Design review of the part built by this model. Coordinates are the model's own, in mm. A direction names the side the tool comes from. Give positions to 0.01 mm unless a question says otherwise; leave off trailing zeros. Write each loop counter-clockwise with the first axis right and the second up, starting at its lowest first coordinate (ties: lowest second). Pieces come first, ordered by that corner, then holes. Notation, with made-up numbers: M 17.5,-5 L 51.5,-5 A8 ccw 51.5,0 Z; hole C 66.25,75 d6. An arc over 180 degrees is marked long. Use a Markdown table: item, result. Add a question column.
```python
from build123d import *

# Parameters (mm, degrees)
SKETCH1_W                = 10
SKETCH1_H                = 20
BOSS_EXTRUDE2_DEPTH      = 10
SKETCH3_W                = 10
SKETCH3_H                = 20
BOSS_EXTRUDE3_DEPTH      = 10
SKETCH4_W                = 62.5
SKETCH4_H                = 5
BOSS_EXTRUDE4_DEPTH      = 10
SKETCH6_R                = 1
CUT_EXTRUDE1_DEPTH       = 10
CUT_EXTRUDE3_START       = -10
SKETCH10_R               = 1
CUT_EXTRUDE3_DEPTH       = 10
SKETCH11_W               = 50
SKETCH11_H               = 50
BOSS_EXTRUDE8_DEPTH      = 10
SKETCH18_W               = 10
SKETCH18_H               = 10
BOSS_EXTRUDE9_DEPTH      = 6
SKETCH20_W               = 10
SKETCH20_H               = 10
BOSS_EXTRUDE10_DEPTH     = 12
SKETCH23_W               = 28.6
SKETCH23_H               = 45
CUT_EXTRUDE10_DEPTH      = 7.5
SKETCH24_W               = 6.4
SKETCH24_H               = 7.5
CUT_EXTRUDE11_DEPTH      = 4.1
SKETCH25_W               = 2.3
SKETCH25_H               = 2.5
CUT_EXTRUDE12_DEPTH      = 41
SKETCH26_W               = 2.3
SKETCH26_H               = 2.4
CUT_EXTRUDE13_DEPTH      = 41
SKETCH27_R               = 1
CUT_EXTRUDE14_DEPTH      = 10
SKETCH28_R               = 1
CUT_EXTRUDE15_DEPTH      = 10
SKETCH31_W               = 12.5
SKETCH31_H               = 10
BOSS_EXTRUDE11_DEPTH     = 5
SKETCH32_W               = 10
SKETCH32_H               = 10
CUT_EXTRUDE16_DEPTH      = 7.5
CUT_EXTRUDE17_DEPTH      = 7.5
SKETCH33_W               = 10
SKETCH33_H               = 10
BOSS_EXTRUDE12_DEPTH     = 5
SKETCH34_W               = 10
SKETCH34_H               = 10
BOSS_EXTRUDE13_DEPTH     = 5
SKETCH35_W               = 10
SKETCH35_H               = 10
BOSS_EXTRUDE14_DEPTH     = 3.5
SKETCH36_W               = 10
SKETCH36_H               = 10
BOSS_EXTRUDE15_DEPTH     = 9.5
CUT_EXTRUDE18_DEPTH      = 90.5
CUT_EXTRUDE18_DEPTH_BACK = 15.5
SKETCH37_R               = 1.25
CUT_EXTRUDE19_DEPTH      = 88.5
CUT_EXTRUDE19_DEPTH_BACK = 15.5
SKETCH38_R               = 1.25
SKETCH39_W               = 29.967126749
SKETCH39_H               = 31.835751001
SKETCH39_W_2             = 15.617210398
SKETCH39_H_2             = 32.298255859
CUT_EXTRUDE20_DEPTH      = 36
SKETCH40_W               = 10
SKETCH40_H               = 50
BOSS_EXTRUDE16_DEPTH     = 11
SKETCH41_W               = 4
SKETCH41_H               = 10
BOSS_EXTRUDE17_DEPTH     = 10
SKETCH42_R               = 1.5
CUT_EXTRUDE21_DEPTH      = 80


with BuildPart() as part:
    # Sketch1 → Boss-Extrude2 (new body)
    with BuildSketch(Plane(origin=(0, 0, 0), x_dir=(1, 0, 0), z_dir=(0, 1, 0))):
        with Locations((5, 10)):
            Rectangle(SKETCH1_W, SKETCH1_H)
    extrude(amount=BOSS_EXTRUDE2_DEPTH)



with BuildPart() as body_2:
    # Sketch3 → Boss-Extrude3 (new body)
    with BuildSketch(Plane(origin=(0, 0, 0), x_dir=(1, 0, 0), z_dir=(0, 1, 0))):
        with Locations((77.5, 10)):
            Rectangle(SKETCH3_W, SKETCH3_H)
    extrude(amount=BOSS_EXTRUDE3_DEPTH)


with BuildPart() as part_1:
    add(part.part)

    add(body_2.part)  # Boss-Extrude4 merges body 2
    # Sketch4 → Boss-Extrude4 (add)
    with BuildSketch(Plane(origin=(0, 0, 0), x_dir=(1, 0, 0), z_dir=(0, 1, 0))):
        with Locations((41.25, 10)):
            Rectangle(SKETCH4_W, SKETCH4_H)
    extrude(amount=BOSS_EXTRUDE4_DEPTH)

    # Sketch6 → Cut-Extrude1 (cut)
    with BuildSketch(Plane(origin=(10, 0, 0), x_dir=(0, 0, -1), z_dir=(1, 0, 0))):
        with Locations((16.25, 5)):
            Circle(SKETCH6_R)
    extrude(amount=-CUT_EXTRUDE1_DEPTH, mode=Mode.SUBTRACT)

    # Sketch10 → Cut-Extrude3 (cut)
    with BuildSketch(Plane.ZY.offset(-72.5).offset(CUT_EXTRUDE3_START)):
        with Locations(Location((-16.25, 5, 0), (0, 0, 180))):
            Circle(SKETCH10_R)
    extrude(amount=CUT_EXTRUDE3_DEPTH, mode=Mode.SUBTRACT)

    # Sketch11 → Boss-Extrude8 (add)
    with BuildSketch(Plane(origin=(0, 0, -12.5), x_dir=(-1, 0, 0), z_dir=(0, 0, -1))):
        with Locations((-35, 20)):
            Rectangle(SKETCH11_W, SKETCH11_H)
    extrude(amount=-BOSS_EXTRUDE8_DEPTH)

    # Sketch18 → Boss-Extrude9 (add)
    with BuildSketch(Plane.XY):
        with Locations((5, 5)):
            Rectangle(SKETCH18_W, SKETCH18_H)
    extrude(amount=BOSS_EXTRUDE9_DEPTH)

    # Sketch20 → Boss-Extrude10 (add)
    with BuildSketch(Plane.XZ):
        with Locations((77.5, -7.5)):
            Rectangle(SKETCH20_W, SKETCH20_H)
        with Locations((5, -7.5)):
            Rectangle(SKETCH20_W, SKETCH20_H)
    extrude(amount=BOSS_EXTRUDE10_DEPTH)

    # Sketch23 → Cut-Extrude10 (cut)
    with BuildSketch(Plane(origin=(0, 0, -12.5), x_dir=(-1, 0, 0), z_dir=(0, 0, -1))):
        with Locations((-35, 22.5)):
            Rectangle(SKETCH23_W, SKETCH23_H)
    extrude(amount=-CUT_EXTRUDE10_DEPTH, mode=Mode.SUBTRACT)

    # Sketch24 → Cut-Extrude11 (cut)
    with BuildSketch(Plane(origin=(0, 45, 0), x_dir=(1, 0, 0), z_dir=(0, 1, 0))):
        with Locations((17.5, 8.75)):
            Rectangle(SKETCH24_W, SKETCH24_H)
        with Locations((52.5, 8.75)):
            Rectangle(SKETCH24_W, SKETCH24_H)
    extrude(amount=-CUT_EXTRUDE11_DEPTH, mode=Mode.SUBTRACT)

    # Sketch25 → Cut-Extrude12 (cut)
    with BuildSketch(Plane(origin=(0, 40.9, 0), x_dir=(1, 0, 0), z_dir=(0, 1, 0))):
        with Locations((50.45, 8.25)):
            Rectangle(SKETCH25_W, SKETCH25_H)
    extrude(amount=-CUT_EXTRUDE12_DEPTH, mode=Mode.SUBTRACT)

    # Sketch26 → Cut-Extrude13 (cut)
    with BuildSketch(Plane(origin=(0, 40.9, 0), x_dir=(1, 0, 0), z_dir=(0, 1, 0))):
        with Locations((19.55, 8.2)):
            Rectangle(SKETCH26_W, SKETCH26_H)
    extrude(amount=-CUT_EXTRUDE13_DEPTH, mode=Mode.SUBTRACT)

    # Sketch27 → Cut-Extrude14 (cut)
    with BuildSketch(Plane(origin=(0, 40.9, 0), x_dir=(1, 0, 0), z_dir=(0, 1, 0))):
        with Locations(Location((17.2, 10.4, 0), (0, 0, 270))):
            Circle(SKETCH27_R)
    extrude(amount=-CUT_EXTRUDE14_DEPTH, mode=Mode.SUBTRACT)

    # Sketch28 → Cut-Extrude15 (cut)
    with BuildSketch(Plane(origin=(0, 40.9, 0), x_dir=(1, 0, 0), z_dir=(0, 1, 0))):
        with Locations(Location((52.8, 10.4, 0), (0, 0, 270))):
            Circle(SKETCH28_R)
    extrude(amount=-CUT_EXTRUDE15_DEPTH, mode=Mode.SUBTRACT)

    # Sketch31 → Boss-Extrude11 (add)
    with BuildSketch(Plane.XY.offset(-7.5)):
        with Locations((66.25, 5)):
            Rectangle(SKETCH31_W, SKETCH31_H)
    extrude(amount=BOSS_EXTRUDE11_DEPTH)

    # Sketch32 → Cut-Extrude16 (cut)
    with BuildSketch(Plane(origin=(0, 0, -20), x_dir=(-1, 0, 0), z_dir=(0, 0, -1))):
        with Locations((-77.5, 5)):
            Rectangle(SKETCH32_W, SKETCH32_H)
    extrude(amount=-CUT_EXTRUDE16_DEPTH, mode=Mode.SUBTRACT)

    # 3DSketch1 → Cut-Extrude17 (cut)
    with BuildSketch(Plane(origin=(10, 0, -20), x_dir=(-0.7071067811865476, 0.7071067811865476, 0), z_dir=(0, 0, 1))):
        Polygon((0, 0), (7.071067812, 7.071067812), (14.142135624, 0), (7.071067812, -7.071067812), align=None)
    extrude(amount=CUT_EXTRUDE17_DEPTH, mode=Mode.SUBTRACT)

    # Sketch33 → Boss-Extrude12 (add)
    with BuildSketch(Plane.XZ.offset(12)):
        with Locations((5, -7.5)):
            Rectangle(SKETCH33_W, SKETCH33_H)
    extrude(amount=BOSS_EXTRUDE12_DEPTH)

    # Sketch34 → Boss-Extrude13 (add)
    with BuildSketch(Plane.XZ.offset(12)):
        with Locations((77.5, -7.5)):
            Rectangle(SKETCH34_W, SKETCH34_H)
    extrude(amount=BOSS_EXTRUDE13_DEPTH)

    # Sketch35 → Boss-Extrude14 (add)
    with BuildSketch(Plane.XY.offset(6)):
        with Locations((5, 5)):
            Rectangle(SKETCH35_W, SKETCH35_H)
    extrude(amount=BOSS_EXTRUDE14_DEPTH)

    # Sketch36 → Boss-Extrude15 (add)
    with BuildSketch(Plane.XY):
        with Locations((77.5, 5)):
            Rectangle(SKETCH36_W, SKETCH36_H)
    extrude(amount=BOSS_EXTRUDE15_DEPTH)

    # Sketch37 → Cut-Extrude18 (cut, two sides: drawn at the far end of the back side and taken through both)
    with BuildSketch(Plane(origin=(10, 0, 0), x_dir=(0, 0, -1), z_dir=(1, 0, 0)).offset(-CUT_EXTRUDE18_DEPTH_BACK)):
        with Locations(Location((-3.5, 5, 0), (0, 0, 180))):
            Circle(SKETCH37_R)
    extrude(amount=CUT_EXTRUDE18_DEPTH + CUT_EXTRUDE18_DEPTH_BACK, mode=Mode.SUBTRACT)

    # Sketch38 → Cut-Extrude19 (cut, two sides: drawn at the far end of the back side and taken through both)
    with BuildSketch(Plane(origin=(10, 0, 0), x_dir=(0, 0, -1), z_dir=(1, 0, 0)).offset(-CUT_EXTRUDE19_DEPTH_BACK)):
        with Locations(Location((7.5, -11, 0), (0, 0, 180))):
            Circle(SKETCH38_R)
    extrude(amount=CUT_EXTRUDE19_DEPTH + CUT_EXTRUDE19_DEPTH_BACK, mode=Mode.SUBTRACT)

    # Sketch39 → Cut-Extrude20 (cut)
    with BuildSketch(Plane(origin=(0, 0, -12.5), x_dir=(-1, 0, 0), z_dir=(0, 0, -1))):
        with Locations((-74.983563375, -4.30748393)):
            Rectangle(SKETCH39_W, SKETCH39_H)
        with Locations((-2.191394801, -3.536642501)):
            Rectangle(SKETCH39_W_2, SKETCH39_H_2)
    extrude(amount=-CUT_EXTRUDE20_DEPTH, mode=Mode.SUBTRACT)

    # Sketch40 → Boss-Extrude16 (add)
    with BuildSketch(Plane(origin=(60, 0, 0), x_dir=(0, 0, -1), z_dir=(1, 0, 0))):
        with Locations((7.5, 20)):
            Rectangle(SKETCH40_W, SKETCH40_H)
    extrude(amount=BOSS_EXTRUDE16_DEPTH)

    # Sketch41 → Boss-Extrude17 (add)
    with BuildSketch(Plane.XY.offset(-2.5)):
        with Locations((12, 40)):
            Rectangle(SKETCH41_W, SKETCH41_H)
        with Locations((12, 0)):
            Rectangle(SKETCH41_W, SKETCH41_H)
        with Locations((69, 40)):
            Rectangle(SKETCH41_W, SKETCH41_H)
        with Locations((69, 0)):
            Rectangle(SKETCH41_W, SKETCH41_H)
    extrude(amount=BOSS_EXTRUDE17_DEPTH)

    # Sketch42 → Cut-Extrude21 (cut)
    with BuildSketch(Plane(origin=(71, 0, 0), x_dir=(0, 0, -1), z_dir=(1, 0, 0))):
        with Locations(Location((-2.5, 0, 0), (0, 0, 90))):
            Circle(SKETCH42_R)
        with Locations(Location((-2.5, 40, 0), (0, 0, 90))):
            Circle(SKETCH42_R)
    extrude(amount=-CUT_EXTRUDE21_DEPTH, mode=Mode.SUBTRACT)


solid = part_1.part
```
(1) Add section C-C on x = 17.2. Give the boundary of the cut face in (y, z).
(2) For pin 1 (2.5 mm diameter, centred on x = 50.5, z = -9, fed in from +Y); pin 2 (1.1 mm diameter, centred on x = 19.5, y = 18, fed in from +Z); pin 3 (1 mm diameter, centred on x = 26, z = -6, fed in from +Y), all flat-tipped, find the tip position at first contact; note any pin that passes through.
(3) Add section B-B on z = 5. Give the boundary of the cut face in (x, y).
(4) Wall thickness on L1, parallel to X at y = 33.5, z = -10.4; L2, parallel to Z at x = 69, y = 40; L3, parallel to Y at x = 68.5, z = -2: over which ranges is each line inside the solid? List them lowest first.
(5) Add section D-D on y = 6.5. Give the boundary of the cut face in (x, z).
(6) Machinability: for faces 4 (the cylindrical face through (52, 36, -11)), 5 (the flat face through (12, 5, 2)), 6 (the flat face through (10, 20, -5)), 7 (the flat face through (69, 40, 7.5)), 8 (the flat face through (35, 0, -9)), which of the approach directions +Z, -Z, +X, -X, +Y, -Y give a long, thin tool a straight path to every point of the face, cutting with its end or side? Answer none if there is none.
(7) The part is to be moulded in two halves that separate along Y. For faces 1 (the cylindrical face through (69, 38.8, 1.6)), 2 (the flat face through (20.7, 20, -11)), 3 (the flat face through (53, 30.9, -10)), say which applies: released by +Y, released by -Y, zero draft, split by the parting line, or undercut.
(8) Add section A-A on y = 40. Give the number of separate pieces and of enclosed holes in the cut face, then the cut area to 3 significant figures.
From the geometry:
| question | item | result |
|---|---|---|
| 1 | outline | M -5,-12.5 L 40.9,-12.5 L 40.9,-11.4 L 30.9,-11.4 L 30.9,-9.4 L 40.9,-9.4 L 40.9,-5 L 45,-5 L 45,-2.5 L -5,-2.5 Z |
| 2 | pin 1 | stops at y = 40.9 |
| 2 | pin 2 | stops at z = -2.5 |
| 2 | pin 3 | stops at y = 0 |
| 3 | outline | M 10,-5 L 14,-5 L 14,5 L 10,5 Z; M 10,35 L 14,35 L 14,45 L 10,45 Z; M 67,-5 L 71,-5 L 71,5 L 67,5 Z; M 67,35 L 71,35 L 71,45 L 67,45 Z |
| 4 | L1 | x = 10 to 16.2, 18.2 to 20.7, 49.3 to 51.8, 53.8 to 71 |
| 4 | L2 | z = -12.5 to 1, 4 to 7.5 |
| 4 | L3 | y = -5 to 5, 35 to 45 |
| 5 | outline | M 10,-12.5 L 20.7,-12.5 L 20.7,-9.4 L 18.4,-9.4 L 18.4,-7 L 20.7,-7 L 20.7,-5 L 49.3,-5 L 49.3,-7 L 51.6,-7 L 51.6,-9.5 L 49.3,-9.5 L 49.3,-12.5 L 71,-12.5 L 71,-2.5 L 10,-2.5 Z |
| 6 | face 4 | +Y |
| 6 | face 5 | +Z, +X, -X |
| 6 | face 6 | +Z, -Z, -X, +Y, -Y |
| 6 | face 7 | +Z, +X, -X, +Y, -Y |
| 6 | face 8 | -Z, +Y |
| 7 | face 1 | undercut |
| 7 | face 2 | zero draft |
| 7 | face 3 | released by +Y |
| 8 | separate pieces | 3 |
| 8 | enclosed holes | 2 |
| 8 | area | 434 mm^2 |
